Model file for the job. Use its own axes, mm. A direction names the side the tool comes from. Give positions to 0.01 mm unless a question says otherwise; leave off trailing zeros. Loops run counter-clockwise (first coordinate to the right, second up) from the corner with the lowest first, then second, coordinate; pieces in that order, holes last. Notation, with made-up numbers: (71.5, -35.75) - (88.5, -35.75) arc R23 cw to (88.5, -25.75) - close; hole circle Ø9 at (-19.75, 28.25). An arc over 180 degrees is marked (long way). Answer as CSV lines item,"result". Start each with the question number.
Item 1: Saw through at D-D on y = -145.5. Give the cut face in (x, z).
Item 2: Drill centre lines: L1, parallel to X at y = -8, z = 38; L2, parallel to X at y = -4, z = -38; L3, parallel to Y at x = 78, z = -39. Where is each one in solid material? Low to high. Write a range as from..to.
Item 3: Pin check, flat tips, straight feed: pin 1 (6.5 mm diameter, centred on x = 65.99, z = 38.1, fed in from -Y); pin 2 (9.5 mm diameter, centred on x = -65.99, z = -38.1, fed in from -Y); pin 3 (4 mm diameter, centred on y = -250.5, z = 19.5, fed in from -X); pin 4 (10 mm diameter, centred on y = -263, z = 58, fed in from +X). Stop position of each tip, or through.
Item 4: Tool access for faces 1 (the flat face through (-43, -6.35, 29)), 2 (the cylindrical face through (-41.45, -6.44, 63.43)): list every direction of +Z, -Z, +X, -X, +Y, -Y with a clear straight run to the whole face (end or side of a thin tool).
Item 5: Saw through at C-C on z = -22. Give the cut face in (x, y), plus the area to 3 significant figures.
Item 6: Saw through at B-B on x = -76.2. Give the cut face in (y, z).
Item 7: Pull direction Z, two halves, no side cores. Call faces 3 (the cylindrical face through (39.01, -6.44, 70.11)), 4 (the cylindrical face through (57.095, -157.575, -2.513)), 5 (the flat face through (41, -12.7, -41)): pulls with the +Z half, pulls with the -Z half, needs draft (parallel to the pull), parting line crosses it, or undercut.
Item 8: Saw through at A-A on z = 0. Give the cut face in (x, y).
from build123d import *

# Parameters (mm, degrees)
F_5_16_CLEARANCE_HOLE1_D = 8.4328
CIRPATTERN1_COUNT        = 12


with BuildPart() as part:
    # Sketch1 → Revolve1 (revolve)
    with BuildSketch(Plane.XY):
        Polygon((-57.15, 0), (-88.9, 0), (-88.9, -12.7), (-57.15, -12.7), (-57.15, -298.45), (-51.1302, -298.45), (-51.1302, -6.35), (-57.15, -6.35), align=None)
    revolve(axis=Axis((0, 0, 0), (0, -1, 0)))

    # 5/16 Clearance Hole1 (through all)
    with Locations(Plane(origin=(0, 0, 0), x_dir=(1, 0, 0), z_dir=(0, 1, 0))):
        with Locations((-76.2, 0)):
            f_5_16_clearance_hole1 = Hole(F_5_16_CLEARANCE_HOLE1_D / 2)

    # CirPattern1: 5/16 Clearance Hole1 ×12 about axis
    cirpattern1_axis = Axis((0, 0, 0), (0, 1, 0))
    for i in range(1, CIRPATTERN1_COUNT):
        add(f_5_16_clearance_hole1.rotate(cirpattern1_axis, i * 360 / CIRPATTERN1_COUNT), mode=Mode.SUBTRACT)


solid = part.part
Responses:
1,outline,"circle Ø114.3 at (0, 0); hole circle Ø102.26 at (0, 0)"
2,L1,"-80.37..-70.21, -61.78..-34.21, 34.21..61.78, 70.21..80.37"
2,L2,"-80.37..-70.21, -61.78..-42.69, 42.69..61.78, 70.21..80.37"
2,L3,"-12.7..0"
3,pin 1,"through"
3,pin 2,"y = -12.7"
3,pin 3,"x = -54.4"
3,pin 4,"x = 21.38"
4,face 1,"+Y"
4,face 2,"+Y, -Y"
5,outline,"(-86.13, -12.7) - (-52.75, -12.7) - (-52.75, -298.45) - (-46.16, -298.45) - (-46.16, -6.35) - (-52.75, -6.35) - (-52.75, 0) - (-86.13, 0) - close; (46.16, -298.45) - (52.75, -298.45) - (52.75, -12.7) - (86.13, -12.7) - (86.13, 0) - (52.75, 0) - (52.75, -6.35) - (46.16, -6.35) - close"
5,area,"4,700 mm2"
6,outline,"(-12.7, -45.79) - (0, -45.79) - (0, -4.22) - (-12.7, -4.22) - close; (-12.7, 4.22) - (0, 4.22) - (0, 45.79) - (-12.7, 45.79) - close"
7,face 3,"undercut"
7,face 4,"parting line crosses it"
7,face 5,"needs draft"
8,outline,"(-88.9, -12.7) - (-80.42, -12.7) - (-80.42, 0) - (-88.9, 0) - close; (-71.98, -12.7) - (-57.15, -12.7) - (-57.15, -298.45) - (-51.13, -298.45) - (-51.13, -6.35) - (-57.15, -6.35) - (-57.15, 0) - (-71.98, 0) - close; (51.13, -298.45) - (57.15, -298.45) - (57.15, -12.7) - (71.98, -12.7) - (71.98, 0) - (57.15, 0) - (57.15, -6.35) - (51.13, -6.35) - close; (80.42, -12.7) - (88.9, -12.7) - (88.9, 0) - (80.42, 0) - close"
